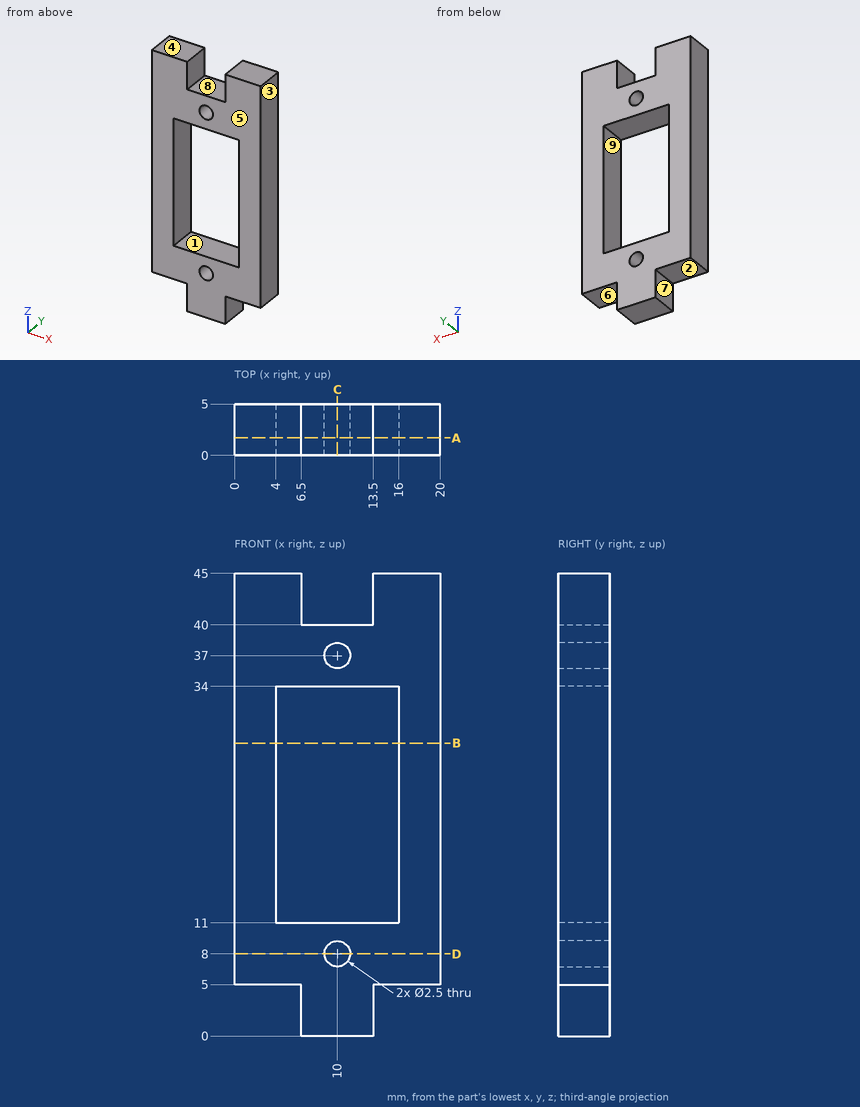
Can you work these out from the drawing? Everything is in mm from the part's minimum corner. A direction names the side the tool comes from. Coordinates: 2 decimals unless noted, no trailing zeros. Write each loop counter-clockwise with the first axis right and the second up, starting at its lowest first coordinate (ties: lowest second). Pieces come first, ordered by that corner, then holes. Notation, with made-up numbers: (63, 45.5) - (74, 45.5) arc R26 cw to (74, 71.5) - close; hole circle Ø3 at (-34.5, -10.5). An arc over 180 degrees is marked (long way). One line per item, written item: value.
1) Suppose I cut it at D-D on z = 8. Write out the boundary of the cut face in (x, y), and give its area (3 significant figures).
Model answer:
outline: (0, 0) - (8.75, 0) - (8.75, 5) - (0, 5) - close; (11.25, 0) - (20, 0) - (20, 5) - (11.25, 5) - close
area: 87.5 mm²
2) We'd pull the mould along Z, two halves only. Please class the marked faces 1, 2, 3 and 4: pulls with the +Z half, pulls with the -Z half, needs draft (parallel to the pull), parting line crosses it, or undercut.
Model answer:
face 1: undercut
face 2: pulls with the -Z half
face 3: needs draft
face 4: pulls with the +Z half
3) On a 3-axis mill with a long thin cutter (end or side, diameter ignored), from which of +Z, -Z, +X, -X, +Y, -Y can I reach the whole of each face in a straight line? I mean the marked faces 5, 6, 7, 8 and 9. Say none if no direction works.
Model answer:
face 5: +Z, -Z, +X, -X, -Y
face 6: -Z, +X, +Y, -Y
face 7: -Z, -X, +Y, -Y
face 8: +Z, +Y, -Y
face 9: +Y, -Y
4) I need wall thicknesses on line 1 along X through (y, z) = (2.6, 8); line 2 along X through (y, z) = (1.4, 43.5); line 3 along Z through (x, y) = (7.75, 3.05). Which ranges of each line are inside material? Lowest first, please.
Model answer:
line 1: x = 0 to 8.75, 11.25 to 20
line 2: x = 0 to 6.5, 13.5 to 20
line 3: z = 0 to 11, 34 to 40
5) Suppose I cut it at B-B on z = 28.5. Write out the boundary of the cut face in (x, y).
Model answer:
outline: (0, 0) - (4, 0) - (4, 5) - (0, 5) - close; (16, 0) - (20, 0) - (20, 5) - (16, 5) - close
6) Suppose I cut it at A-A on y = 1.7. Write out the boundary of the cut face in (x, z), and give its area (3 significant figures).
Model answer:
outline: (0, 5) - (6.5, 5) - (6.5, 0) - (13.5, 0) - (13.5, 5) - (20, 5) - (20, 45) - (13.5, 45) - (13.5, 40) - (6.5, 40) - (6.5, 45) - (0, 45) - close; hole (4, 11) - (16, 11) - (16, 34) - (4, 34) - close; hole circle Ø2.5 at (10, 8); hole circle Ø2.5 at (10, 37)
area: 514 mm²
7) Suppose I cut it at C-C on x = 10. Write out the boundary of the cut face in (y, z), and give its area (3 significant figures).
Model answer:
outline: (0, 0) - (5, 0) - (5, 6.75) - (0, 6.75) - close; (0, 9.25) - (5, 9.25) - (5, 11) - (0, 11) - close; (0, 34) - (5, 34) - (5, 35.75) - (0, 35.75) - close; (0, 38.25) - (5, 38.25) - (5, 40) - (0, 40) - close
area: 60.0 mm²
8) I'm going to push flat-ended pins straight in: P1, Ø2.5, axis at y = 2, z = 3, coming from the +X side; P2, Ø1.5, axis at x = 10, y = 1.5, coming from the +Z side; P3, Ø1.5, axis at x = 2.5, y = 3.5, coming from the -Z side. Where does each tip first touch, or does it pass through?
Model answer:
P1: stops at x = 13.5
P2: stops at z = 40
P3: stops at z = 5
